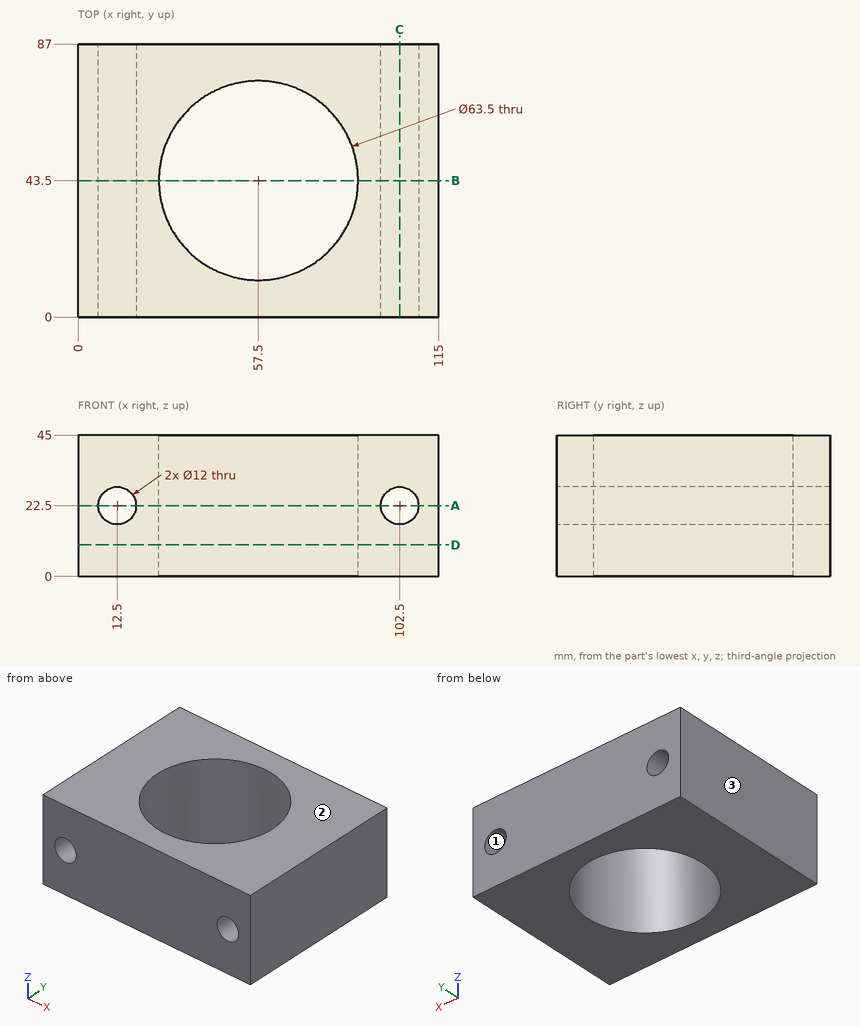
Here's the drawing with two shaded views (mm, measured from the low corner). I have some questions. Coordinates: 2 decimals unless noted, no trailing zeros. Write each loop counter-clockwise with the first axis right and the second up, starting at its lowest first coordinate (ties: lowest second). Pieces come first, ordered by that corner, then holes. Notation, with made-up numbers: (-22.5, 62) -> (26.5, 62) arc R21 cw to (26.5, 100) -> close; hole circle Ø1 at (32, 29). An arc over 180 degrees is marked (long way). One line per question, with ' | ' between items. Start each with the question number.
1. Please list where these lines run through material, in increasing order: line 1 along Z through (x, y) = (12.5, 35); line 2 along X through (y, z) = (30, 22); line 3 along Y through (x, z) = (57, 19).
2. If we section it at C-C (x = 102.5): Please give me the cut outline in (y, z).
3. Thinking about a two-plate mould opening in X: for the marked faces 1, 2 and 3, which applies, pulls with the +X half, pulls with the -X half, needs draft (parallel to the pull), parting line crosses it, or undercut?
4. If we section it at A-A (z = 22.5): Please give me the cut outline in (x, y).
5. If we section it at D-D (z = 10): Please give me the cut outline in (x, y), and give its area (3 significant figures).
6. If we section it at B-B (y = 43.5): Please give me the cut outline in (x, z), and give its area (3 significant figures).
Return value:
1) line 1: z = 0 to 16.5, 28.5 to 45 | line 2: x = 0 to 6.52, 18.48 to 28.76, 86.24 to 96.52, 108.48 to 115 | line 3: y = 0 to 11.75, 75.25 to 87
2) outline: (0, 0) -> (87, 0) -> (87, 16.5) -> (0, 16.5) -> close; (0, 28.5) -> (87, 28.5) -> (87, 45) -> (0, 45) -> close
3) face 1: undercut | face 2: needs draft | face 3: pulls with the -X half
4) outline: (0, 0) -> (6.5, 0) -> (6.5, 87) -> (0, 87) -> close; (18.5, 0) -> (96.5, 0) -> (96.5, 87) -> (18.5, 87) -> close; (108.5, 0) -> (115, 0) -> (115, 87) -> (108.5, 87) -> close; hole circle Ø63.5 at (57.5, 43.5)
5) outline: (0, 0) -> (115, 0) -> (115, 87) -> (0, 87) -> close; hole circle Ø63.5 at (57.5, 43.5) | area: 6,840 mm²
6) outline: (0, 0) -> (25.75, 0) -> (25.75, 45) -> (0, 45) -> close; (89.25, 0) -> (115, 0) -> (115, 45) -> (89.25, 45) -> close; hole circle Ø12 at (12.5, 22.5); hole circle Ø12 at (102.5, 22.5) | area: 2,090 mm²
